Verification items for the finished model (mm, model axes). Face numbers are marked on the shaded views. A direction names the side the tool comes from. Give positions to 0.01 mm unless a question says otherwise; leave off trailing zeros. Write each loop counter-clockwise with the first axis right and the second up, starting at its lowest first coordinate (ties: lowest second). Pieces come first, ordered by that corner, then holes. Notation, with made-up numbers: (40.25, -24.5) -> (47.25, -24.5) arc R20 cw to (47.25, 0.5) -> close; hole circle Ø5 at (61.5, 87). An arc over 180 degrees is marked (long way). Use one line per item in the form item = value. Start each with the question number.
(1) Section check A-A, the plane z = 3.9. Record the cut outline in (x, y).
(2) Section check D-D, the plane z = 1.5. Record the cut outline in (x, y).
(3) Scan lines: L1, parallel to X at y = -4.5, z = 3; L2, parallel to X at y = -21.25, z = 3.5; L3, parallel to Y at x = -18.75, z = 6. Record each from-to range of solid material in increasing order.
(4) Section check B-B, the plane y = -4. Record the cut outline in (x, z).
(5) Set-up check for the marked faces 4, 5 and 6: record each of +Z, -Z, +X, -X, +Y, -Y from which the full face is reachable in a straight line by a thin tool's end or side.
(6) Section check C-C, the plane x = -12. Record the cut outline in (y, z).
(7) Depth check by flat-ended pin: pin 1 Ø0.9 at (x, z) = (-18.5, 3) entering from -Y; pin 2 Ø3 at (x, y) = (-14.5, -6.5) entering from +Z; pin 3 Ø2.5 at (y, z) = (-13, 4.5) entering from -X. Enter the tip coordinate at first touch or a pass-through.
(8) Release check for a two-part mould opening along X. For the marked faces 1, 2 and 3 record: pulls with the +X half, pulls with the -X half, needs draft (parallel to the pull), parting line crosses it, or undercut.
from build123d import *

# Parameters (mm, degrees)
PAD_DEPTH       = 7.8
SKETCH001_R     = 1.85
POCKET_DEPTH    = 5
CHAMFER_SIZE    = 0.5
CHAMFER001_SIZE = 1
FILLET_R        = 2


with BuildPart() as part:
    # Sketch → Pad (new body)
    with BuildSketch(Plane.XY):
        Polygon((-16.794462, -6.264032), (-19.594462, -6.264032), (-19.594462, 0.735968), (-8.544462, 0.735968), (-8.544462, -23.264032), (-12.544462, -23.264032), (-12.544462, -3.264032), (-16.794462, -3.264032), align=None)
    extrude(amount=PAD_DEPTH)

    # Sketch001 (on Face4 of Pad) → Pocket (cut)
    with BuildSketch(Plane.YZ.offset(-8.544462)):
        with Locations((-18.264032, 3.9)):
            Circle(SKETCH001_R)
    extrude(amount=-POCKET_DEPTH, mode=Mode.SUBTRACT)

    # Chamfer
    chamfer_edges = [part.edges().sort_by_distance(p)[0] for p in [
        (-16.794462, -6.264032, 3.9),
        (-18.194462, -6.264032, 0),
        (-19.594462, -6.264032, 3.9),
        (-18.194462, -6.264032, 7.8),
    ]]
    chamfer(chamfer_edges, length=CHAMFER_SIZE)

    # Chamfer001
    chamfer001_edges = [part.edges().sort_by_distance(p)[0] for p in [
        (-8.544462, -23.264032, 3.9),
    ]]
    chamfer(chamfer001_edges, length=CHAMFER001_SIZE)

    # Fillet
    fillet_edges = [part.edges().sort_by_distance(p)[0] for p in [
        (-8.544462, 0.735968, 3.9),
    ]]
    fillet(fillet_edges, radius=FILLET_R)


solid = part.part
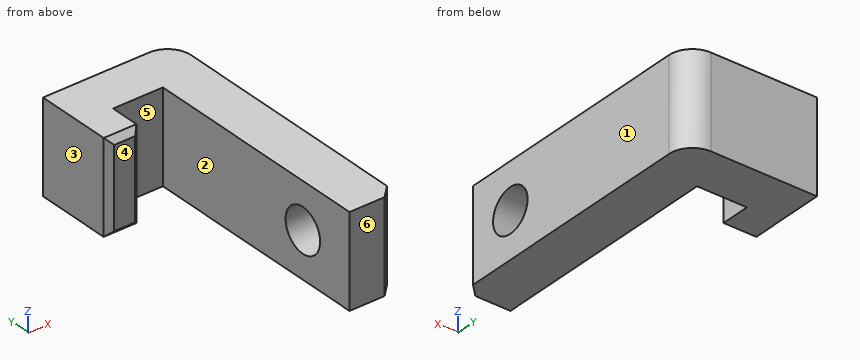
Completed:
q1.outline = (-19.59, -5.76) -> (-19.09, -6.26) -> (-17.29, -6.26) -> (-16.79, -5.76) -> (-16.79, -3.26) -> (-12.54, -3.26) -> (-12.54, -16.41) -> (-8.54, -16.41) -> (-8.54, -1.26) arc R2 ccw to (-10.54, 0.74) -> (-19.59, 0.74) -> close; (-12.54, -23.26) -> (-9.54, -23.26) -> (-8.54, -22.26) -> (-8.54, -20.11) -> (-12.54, -20.11) -> close
q2.outline = (-19.59, -5.76) -> (-19.09, -6.26) -> (-17.29, -6.26) -> (-16.79, -5.76) -> (-16.79, -3.26) -> (-12.54, -3.26) -> (-12.54, -23.26) -> (-9.54, -23.26) -> (-8.54, -22.26) -> (-8.54, -1.26) arc R2 ccw to (-10.54, 0.74) -> (-19.59, 0.74) -> close
q3.L1 = -19.59 to -16.79, -12.54 to -8.54
q3.L2 = -12.54 to -8.54
q3.L3 = -6.26 to 0.74
q4.outline = (-19.59, 0) -> (-16.79, 0) -> (-16.79, 7.8) -> (-19.59, 7.8) -> close; (-12.54, 0) -> (-8.54, 0) -> (-8.54, 7.8) -> (-12.54, 7.8) -> close
q5.face_4 = +Z, -Z, -X, -Y
q5.face_5 = +Z, -Z, -Y
q5.face_6 = +Z, -Z, +X, -X, -Y
q6.outline = (-23.26, 0) -> (0.74, 0) -> (0.74, 7.8) -> (-23.26, 7.8) -> close; hole circle Ø3.7 at (-18.26, 3.9)
q7.pin_1 = -6.26
q7.pin_2 = through
q7.pin_3 = -12.54
q8.face_1 = pulls with the +X half
q8.face_2 = undercut
q8.face_3 = pulls with the -X half
